Autodesk Inventor part; units mm, degrees
ref_plane "YZ Plane" through (0, 0, 0) normal (1, 0, 0) x (0, 1, 0)
ref_plane "XZ Plane" through (0, 0, 0) normal (0, 1, 0) x (-1, 0, 0)
ref_plane "XY Plane" through (0, 0, 0) normal (0, 0, 1) x (1, 0, 0)
sketch "Sketch1" plane through (0, 0, 0) normal (0, 0, 1) x (1, 0, 0)
  arc A0 (17.969, 11.935) -> (18.35, 12.316) centre (17.969, 12.316) ccw
  line L0 (13.205, 11.935) -> (17.969, 11.935)
  arc A1 (11.935, 13.205) -> (13.205, 11.935) centre (13.205, 13.205) ccw
  line L1 (11.935, 17.969) -> (11.935, 13.205)
  arc A2 (12.316, 18.35) -> (11.935, 17.969) centre (12.316, 17.969) ccw
  line L2 (15.556, 18.35) -> (12.316, 18.35)
  arc A3 (18.35, 15.556) -> (15.556, 18.35) centre (15.556, 15.556) ccw
  line L3 (18.35, 12.316) -> (18.35, 15.556)
  circle A4 centre (0, 0) radius 3.4
  arc A5 (-9.0762, -5.7416) -> (-7.685, -2.3829) centre (-12.4348, -2.3829) ccw
  line L4 (-11.6227, -8.288) -> (-9.0762, -5.7416)
  arc A6 (-11.6227, -8.288) -> (-11.8458, -8.8268) centre (-11.0838, -8.8268) ccw
  line L5 (-11.8458, -9.1968) -> (-11.8458, -8.8268)
  arc A7 (-12.069, -9.7356) -> (-11.8458, -9.1968) centre (-12.6078, -9.1968) ccw
  line L6 (-17.924, -15.5906) -> (-12.069, -9.7356)
  arc A8 (-18.35, -15.4141) -> (-17.924, -15.5906) centre (-18.1005, -15.4141) ccw
  line L7 (-18.35, 15.541) -> (-18.35, -15.4141)
  arc A9 (-15.556, 18.335) -> (-18.35, 15.541) centre (-15.556, 15.541) ccw
  line L8 (-12.316, 18.335) -> (-15.556, 18.335)
  arc A10 (-11.935, 17.954) -> (-12.316, 18.335) centre (-12.316, 17.954) ccw
  line L9 (-11.935, 9.7626) -> (-11.935, 17.954)
  arc A11 (-11.935, 9.7626) -> (-11.0051, 7.5175) centre (-8.76, 9.7626) ccw
  line L10 (-9.0762, 5.5886) -> (-11.0051, 7.5175)
  arc A12 (-7.685, 2.23) -> (-9.0762, 5.5886) centre (-12.4348, 2.23) ccw
  line L11 (-7.685, -2.3829) -> (-7.685, 2.23)
  line L12 (-15.4141, -18.35) -> (15.556, -18.35)
  arc A13 (-15.5906, -17.924) -> (-15.4141, -18.35) centre (-15.4141, -18.1005) ccw
  line L13 (-9.8056, -12.139) -> (-15.5906, -17.924)
  arc A14 (-9.2667, -11.9158) -> (-9.8056, -12.139) centre (-9.2667, -12.6778) ccw
  line L14 (-8.8204, -11.9158) -> (-9.2667, -11.9158)
  arc A15 (-8.8204, -11.9158) -> (-8.2816, -11.6926) centre (-8.8204, -11.1538) ccw
  line L15 (-5.6501, -9.0612) -> (-8.2816, -11.6926)
  arc A16 (-2.2915, -7.67) -> (-5.6501, -9.0612) centre (-2.2915, -12.4198) ccw
  line L16 (3.3048, -7.67) -> (-2.2915, -7.67)
  arc A17 (6.6634, -9.0612) -> (3.3048, -7.67) centre (3.3048, -12.4198) ccw
  line L17 (8.6072, -11.0051) -> (6.6634, -9.0612)
  arc A18 (8.6072, -11.0051) -> (10.8523, -11.935) centre (10.8523, -8.76) ccw
  line L18 (17.8551, -11.935) -> (10.8523, -11.935)
  arc A19 (18.35, -12.4299) -> (17.8551, -11.935) centre (17.8551, -12.4299) ccw
  line L19 (18.35, -15.556) -> (18.35, -12.4299)
  arc A20 (15.556, -18.35) -> (18.35, -15.556) centre (15.556, -15.556) ccw
  line L20 (-16.825, -20) -> (16.825, -20)
  arc A21 (16.825, -20) -> (20, -16.825) centre (16.825, -16.825) ccw
  line L21 (20, -16.825) -> (20, -5.6348)
  arc A22 (20, -5.6348) -> (18.4252, -4.06) centre (18.4252, -5.6348) ccw
  line L22 (18.4252, -4.06) -> (17.5148, -4.06)
  arc A23 (17.5148, -4.06) -> (15.94, -5.6348) centre (17.5148, -5.6348) ccw
  line L23 (15.94, -5.6348) -> (15.94, -6.8785)
  line L24 (15.94, -6.8785) -> (16.7025, -6.8785)
  line L25 (16.7025, -6.8785) -> (16.7025, -9.015)
  arc A24 (15.4325, -10.285) -> (16.7025, -9.015) centre (15.4325, -9.015) ccw
  line L26 (15.4325, -10.285) -> (12.4956, -10.285)
  arc A25 (11.867, -10.0246) -> (12.4956, -10.285) centre (12.4956, -9.396) ccw
  line L27 (11.867, -10.0246) -> (9.0762, -7.2338)
  arc A26 (7.685, -3.8752) -> (9.0762, -7.2338) centre (12.4348, -3.8752) ccw
  line L28 (7.685, -3.8752) -> (7.685, 2.341)
  arc A27 (9.0762, 5.6996) -> (7.685, 2.341) centre (12.4348, 2.341) ccw
  line L29 (9.0762, 5.6996) -> (13.4012, 10.0246)
  arc A28 (14.0298, 10.285) -> (13.4012, 10.0246) centre (14.0298, 9.396) ccw
  line L30 (14.0298, 10.285) -> (15.432, 10.285)
  arc A29 (16.702, 9.015) -> (15.432, 10.285) centre (15.432, 9.015) ccw
  line L31 (16.702, 9.015) -> (16.702, 6.8785)
  line L32 (16.702, 6.8785) -> (15.94, 6.8785)
  line L33 (15.94, 6.8785) -> (15.94, 5.6348)
  arc A30 (15.94, 5.6348) -> (17.5148, 4.06) centre (17.5148, 5.6348) ccw
  line L34 (17.5148, 4.06) -> (18.4252, 4.06)
  arc A31 (18.4252, 4.06) -> (20, 5.6348) centre (18.4252, 5.6348) ccw
  line L35 (20, 5.6348) -> (20, 16.825)
  arc A32 (20, 16.825) -> (16.825, 20) centre (16.825, 16.825) ccw
  line L36 (16.825, 20) -> (5.6348, 20)
  arc A33 (5.6348, 20) -> (4.06, 18.4252) centre (5.6348, 18.4252) ccw
  line L37 (4.06, 18.4252) -> (4.06, 17.5148)
  arc A34 (4.06, 17.5148) -> (5.6348, 15.94) centre (5.6348, 17.5148) ccw
  line L38 (5.6348, 15.94) -> (6.8785, 15.94)
  line L39 (6.8785, 15.94) -> (6.8785, 16.7025)
  line L40 (6.8785, 16.7025) -> (9.015, 16.7025)
  arc A35 (10.285, 15.4325) -> (9.015, 16.7025) centre (9.015, 15.4325) ccw
  line L41 (10.285, 15.4325) -> (10.285, 14.0298)
  arc A36 (10.0246, 13.4012) -> (10.285, 14.0298) centre (9.396, 14.0298) ccw
  line L42 (10.0246, 13.4012) -> (5.7146, 9.0912)
  arc A37 (2.356, 7.7) -> (5.7146, 9.0912) centre (2.356, 12.4498) ccw
  line L43 (2.356, 7.7) -> (-2.356, 7.7)
  arc A38 (-5.7146, 9.0912) -> (-2.356, 7.7) centre (-2.356, 12.4498) ccw
  line L44 (-5.7146, 9.0912) -> (-10.0246, 13.4012)
  arc A39 (-10.285, 14.0298) -> (-10.0246, 13.4012) centre (-9.396, 14.0298) ccw
  line L45 (-10.285, 14.0298) -> (-10.285, 15.4325)
  arc A40 (-9.015, 16.7025) -> (-10.285, 15.4325) centre (-9.015, 15.4325) ccw
  line L46 (-9.015, 16.7025) -> (-6.8785, 16.7025)
  line L47 (-6.8785, 16.7025) -> (-6.8785, 15.94)
  line L48 (-6.8785, 15.94) -> (-5.6348, 15.94)
  arc A41 (-5.6348, 15.94) -> (-4.06, 17.5148) centre (-5.6348, 17.5148) ccw
  line L49 (-4.06, 17.5148) -> (-4.06, 18.4252)
  arc A42 (-4.06, 18.4252) -> (-5.6348, 20) centre (-5.6348, 18.4252) ccw
  line L50 (-5.6348, 20) -> (-16.825, 20)
  arc A43 (-16.825, 20) -> (-20, 16.825) centre (-16.825, 16.825) ccw
  line L51 (-20, 16.825) -> (-20, -16.825)
  arc A44 (-20, -16.825) -> (-16.825, -20) centre (-16.825, -16.825) ccw
extrude "Extrusion1" add sketch "Sketch1" against normal blind 100
properties part number "40-4002-BLACK-FB"
Source: CAD feature listing. Evaluate the final solid. Frame: model axes, mm. A direction names the side the tool comes from. Coordinates: 2 decimals unless noted, no trailing zeros. Loops run counter-clockwise (first coordinate to the right, second up) from the corner with the lowest first, then second, coordinate; pieces in that order, holes last. Notation, with made-up numbers: (20, 34.5) - (35, 34.5) arc R11 ccw to (35, 38.5) - close; hole circle Ø3 at (62.5, 70). An arc over 180 degrees is marked (long way). Return JSON: item names as keys, results as strings.
Q1. Section A-A, the plane x = 0. Return loops of the section in (y, z), plus the area to 3 significant figures.
Results:
{"outline": "(-20, -100) - (-18.35, -100) - (-18.35, 0) - (-20, 0) - close; (-7.67, -100) - (-3.4, -100) - (-3.4, 0) - (-7.67, 0) - close; (3.4, -100) - (7.7, -100) - (7.7, 0) - (3.4, 0) - close", "area": "1,020 mm2"}
Q2. Contact query for flat-ended pins moving along their axis: P1, Ø8, axis at y = -1.5, z = -72.5, coming from the +X side; P2, Ø1, axis at y = 18, z = -73, coming from the +X side. Output: stop coordinate, or through.
Results:
{"P1": "x = 19.99", "P2": "x = 19.93"}
Q3. Section B-B, the plane y = 0. Return loops of the section in (x, z) (3 decimals).
Results:
{"outline": "(-20, -100) - (-18.35, -100) - (-18.35, 0) - (-20, 0) - close; (-7.685, -100) - (-3.4, -100) - (-3.4, 0) - (-7.685, 0) - close; (3.4, -100) - (7.685, -100) - (7.685, 0) - (3.4, 0) - close"}
Q4. Access query for faces 5 (the flat face through (10.49, -8.65, -49.3)), 6 (the flat face through (-20, 0, -49)), 7 (the flat face through (7.685, -1, -49)), 8 (the flat face through (0, 7.7, -49)), 9 (the flat face through (1, 5, -100)). Directions: +Z, -Z, +X, -X, +Y, -Y. A direction counts if a zero-diameter tool reaches every point of the face in a straight line with its end or side. Return the directions, or none.
Results:
{"face 5": "+Z, -Z", "face 6": "+Z, -Z, -X, +Y, -Y", "face 7": "+Z, -Z, +X", "face 8": "+Z, -Z, +Y", "face 9": "-Z, +X, -X, +Y, -Y"}
Q5. Mould query, pull axis X, two halves, no side actions, for faces 1 (the flat face through (0, -20, -49)), 2 (the cylindrical face through (19.05, -19.09, -49.3)), 3 (the flat face through (1, -7.67, -49)), 4 (the flat face through (-15.037, -12.704, -49.3)). Classes: released by +X, released by -X, zero draft, split by the parting line, or undercut.
Results:
{"face 1": "zero draft", "face 2": "released by +X", "face 3": "undercut", "face 4": "undercut"}
Q6. Material intervals for line 1 along Y through (x, z) = (0, -43); line 2 along X through (y, z) = (-10, -19); line 3 along X through (y, z) = (6, -44), sorted ascending.
Results:
{"line 1": "-20 to -18.35, -7.67 to -3.4, 3.4 to 7.7", "line 2": "-20 to -18.35, -12.33 to -6.59, 7.6 to 11.84, 16.23 to 20", "line 3": "-20 to -18.35, -9.49 to 9.38, 15.94 to 20"}
Q7. Section C-C, the plane z = -75. Give the number of separate pieces and of enclosed holes in the cut face, plus the area to 3 significant figures.
Results:
{"separate pieces": "1", "enclosed holes": "4", "area": "655 mm2"}
